Autodesk Inventor part; units mm, degrees
ref_plane "Work Plane2" through (-30, -30, 6) normal (0, 0, -1) x (0, 1, 0)
ref_plane "YZ Plane" through (0, 0, 0) normal (1, 0, 0) x (0, 1, 0)
ref_plane "XZ Plane" through (0, 0, 0) normal (0, 1, 0) x (-1, 0, 0)
ref_plane "Work Plane1" through (0, 0, 0) normal (0, 0, 1) x (1, 0, 0)
ref_plane "Work Plane2" through (-30, -30, 6) normal (0, 0, -1) x (0, 1, 0)
sketch "Sketch1" plane through (0, 0, 0) normal (0, 0, 1) x (1, 0, 0)
  circle A0 centre (-25, 0) radius 1.95
  circle A1 centre (0, -25) radius 1.95
  circle A2 centre (25, -25) radius 1.95
  circle A3 centre (-25, 25) radius 1.95
  circle A4 centre (25, 25) radius 1.95
  circle A5 centre (-25, -25) radius 1.95
  circle A6 centre (0, 25) radius 1.95
  circle A7 centre (25, 0) radius 1.95
  line L0 (-30, -28) -> (-28, -30)
  line L1 (-28, -30) -> (28, -30)
  line L2 (28, -30) -> (30, -28)
  line L3 (30, -28) -> (30, 28)
  line L4 (30, 28) -> (28, 30)
  line L5 (28, 30) -> (-28, 30)
  line L6 (-28, 30) -> (-30, 28)
  line L7 (-30, 28) -> (-30, -28)
  line L8 (43, -44) -> (44, -44)
  line L9 (76, -44) -> (145, -44) construction
  point P0 (0, 0)
  point P1 (30, 25)
extrude "Extrusion1" add sketch "Sketch1" along normal up to surface (6 mm away) contours A0 | A1 | A2 | A3 | A4 | A5 | A6 | A7 | L7 L6 L5 L4 L3 L2 L1 L0
sketch "Sketch2" plane through (-28, 30, 6) normal (0, 0, 1) x (1, 0, 0)
  circle A0 centre (10.5, -12.5) radius 1.95
  circle A1 centre (10.5, -47.5) radius 1.95
  circle A2 centre (45.5, -47.5) radius 1.95
  circle A3 centre (45.5, -12.5) radius 1.95
  point P0 (28, -30)
hole "Hole1" at (-17.5, -17.5, 6) at (17.5, -17.5, 6) at (17.5, 17.5, 6) at (-17.5, 17.5, 6) direction (0, 0, -1) diameter 4 end through all counterbore diameter 8 counterbore depth 4.5
sketch "Sketch10" plane through (0, 0, 0) normal (0, 0, -1) x (-1, 0, 0)
  circle A0 centre (-25, 25) radius 2.325
  circle A1 centre (-25, -25) radius 2.325
  circle A2 centre (25, 25) radius 2.325
  circle A3 centre (25, -25) radius 2.325
  circle A4 centre (25, -25) radius 2.325
  point P0 (0, 0)
hole "Hole3" at (-25, 25, 0) at (25, 25, 0) at (-25, -25, 0) at (25, -25, 0) direction (0, 0, 1) diameter 3.8 depth 20 tip angle 118
sketch "Skizze13" plane through (30, -28, 0) normal (1, 0, 0) x (0, 0, -1)
  line L0 (0, 56) -> (-6, 56)
  line L1 (-6, 56) -> (-6, 58)
  line L2 (0, 56) -> (0, 58)
  line L3 (0, 58) -> (-6, 58)
  line L4 (-6, 58) -> (-6, 63)
  line L5 (-6, 63) -> (6.4834, 75.4834)
  line L6 (10.5521, 75.4834) -> (12.5521, 75.4834)
  line L7 (0, 58) -> (0, 61)
  line L8 (0, 61) -> (8.4834, 69.4834)
  line L9 (8.4834, 69.4834) -> (42.5521, 69.4834)
  line L10 (42.5521, 69.4834) -> (42.5521, 75.4834)
  line L11 (42.5521, 75.4834) -> (6.4834, 75.4834)
  line L12 (42.5521, 75.4834) -> (42.5521, 107.4834)
  point P0 (0, 28)
  dimension "d43" = 5
  dimension "d44" = 135
  dimension "d45" = 135
  dimension "d46" = 0
  dimension "d49" = 6
extrude "Extrusion10" add sketch "Skizze13" against normal up to surface (60 mm away)
ref_plane "Arbeitsebene4" through (-30, 57.7593, -26.2973) normal (1, 0, 0) x (0, -0.9086751, 0.417504)
sketch "Skizze14" plane through (-30, -28, 0) normal (-1, 0, 0) x (0, 0, 1)
  circle A0 centre (-16.0521, 80.4834) radius 1
  circle A1 centre (-31.5521, 101.9834) radius 1
  circle A2 centre (-36.5521, 73.9834) radius 1
  line L0 (-6.4834, 75.4834) -> (-42.5521, 75.4834)
  line L1 (-42.5521, 69.4834) -> (-42.5521, 75.4834)
  line L2 (-42.5521, 75.4834) -> (-12.5521, 75.4834)
  line L3 (-12.5521, 75.4834) -> (-12.5521, 105.4834)
  line L4 (-12.5521, 105.4834) -> (-42.5521, 105.4834)
  line L5 (-42.5521, 105.4834) -> (-42.5521, 75.4834)
  circle A3 centre (-26.5521, 91.4834) radius 2.6486
  line L6 (-34.0521, 83.9834) -> (-19.0521, 83.9834)
  line L7 (-19.0521, 83.9834) -> (-19.0521, 98.9834)
  line L8 (-19.0521, 98.9834) -> (-34.0521, 98.9834)
  line L9 (-34.0521, 98.9834) -> (-34.0521, 83.9834)
  line L10 (-34.0521, 83.9834) -> (-19.0521, 98.9834) construction
  line L11 (-19.0521, 83.9834) -> (-34.0521, 98.9834) construction
  point P0 (0, 28)
  point P1 (-12.5521, 75.4834)
  dimension "d50" = 30
  dimension "d51" = 30
  dimension "d52" = 15
  dimension "d53" = 15
extrude "Extrusion11" add sketch "Skizze14" against normal blind 5 contours L0 L5 L4 L3
sketch "Skizze15" plane through (30, 47.4834, -6.4834) normal (0, 1, 0) x (1, 0, 0)
  circle A0 centre (-15, 20.0687) radius 1.4
  line L0 (2.6067, 20.0687) -> (-28.3951, 20.0687) construction
  line L1 (2.6067, 21.6687) -> (-28.3951, 21.6687)
  line L2 (-28.3951, 18.4687) -> (2.6067, 18.4687)
  arc A1 (2.6067, 18.4687) -> (2.6067, 21.6687) centre (2.6067, 20.0687) ccw
  arc A2 (-28.3951, 21.6687) -> (-28.3951, 18.4687) centre (-28.3951, 20.0687) ccw
  point P0 (-30, -6.4834)
  point P1 (-12.8942, 20.0687)
  dimension "d56" = 3.2
extrude "Extrusion12" cut sketch "Skizze15" against normal through all contours A0 | A1 L2 A2 L1
sketch "Skizze16" plane through (-30, -28, 0) normal (-1, 0, 0) x (0, 0, 1)
  circle A0 centre (-16.0521, 80.4834) radius 1
  circle A1 centre (-31.5521, 101.9834) radius 1
  circle A2 centre (-36.5521, 73.9834) radius 1
  point P0 (0, 28)
extrude "Extrusion13" cut sketch "Skizze16" against normal blind 10
sketch "Skizze17" plane through (-30, 47.4834, -6.4834) normal (0, 1, 0) x (1, 0, 0)
  arc A0 (31.6049, 21.6687) -> (31.6049, 18.4687) centre (31.6049, 20.0687) ccw
  line L0 (44.28, 10.0687) -> (26.9595, 20.0687)
  line L1 (26.9595, 20.0687) -> (44.28, 30.0687)
  line L2 (44.28, 30.0687) -> (44.28, 10.0687)
  line L3 (0, 6.0687) -> (0, 36.0687)
  point P0 (30, -6.4834)
  point P1 (38.5065, 20.0687)
  dimension "d61" = 20
hole "Bohrung4" at (14.28, 47.4834, -16.5521) at (-3.0405, 47.4834, -26.5521) at (14.28, 47.4834, -36.5521) direction (0, -1, 0) diameter 2.8 depth 20 tip angle 118
properties part number "cellSTORM_v5_laserstage"
Could you check a few things on this model? Use its own coordinates, in mm. A direction names the side the tool comes from. Coordinates: 2 decimals unless noted, no trailing zeros. Loops run counter-clockwise (first coordinate to the right, second up) from the corner with the lowest first, then second, coordinate; pieces in that order, holes last.
1) Imagine slicing it at A-A (y = -17.5). List the corners of the cut face in (x, z) for me.
Reported:
outline: (-30, 0) - (-19.5, 0) - (-19.5, 1.5) - (-21.5, 1.5) - (-21.5, 6) - (-30, 6) - close; (-15.5, 0) - (15.5, 0) - (15.5, 1.5) - (13.5, 1.5) - (13.5, 6) - (-13.5, 6) - (-13.5, 1.5) - (-15.5, 1.5) - close; (19.5, 0) - (30, 0) - (30, 6) - (21.5, 6) - (21.5, 1.5) - (19.5, 1.5) - close
2) Which directions (+Z, -Z, +X, -X, +Y, -Y) give clear straight access to the entire face, cutting with the end or side of a thin tool? Please do faces 5 (the face through (-15.8, 15.8, 1.5)), 6 (the face through (-28, 70.983, -26)), 7 (the face through (-28, 62, -12.552)), 8 (the face through (-30, 45, -18)).
Reported:
face 5: +Z
face 6: +X, -X
face 7: +Z, +X, -X, +Y
face 8: +Z, -Z, -X, +Y, -Y
3) Imagine slicing it at D-D (y = 62). List the corners of the cut face in (x, z) for me.
Reported:
outline: (-30, -42.55) - (-25, -42.55) - (-25, -34.05) - (-30, -34.05) - close; (-30, -19.05) - (-25, -19.05) - (-25, -12.55) - (-30, -12.55) - close
4) Thinking about a two-plate mould opening in Y: for faces 1 (the face through (30, 44, -35)), 2 (the face through (15.517, -17.24, 0.74)), 3 (the face through (0, 41, 0)), 4 (the face through (14.8, -14.55, 3.72)), which applies, released by +Y, released by -Y, zero draft, split by the parting line, or undercut?
Reported:
face 1: zero draft
face 2: undercut
face 3: released by +Y
face 4: undercut
5) Imagine slicing it at C-C (x = -17.5). List the corners of the cut face in (y, z) for me, and give its area (3 significant figures).
Reported:
outline: (-30, 0) - (-19.5, 0) - (-19.5, 1.5) - (-21.5, 1.5) - (-21.5, 6) - (-30, 6) - close; (-15.5, 0) - (15.5, 0) - (15.5, 1.5) - (13.5, 1.5) - (13.5, 6) - (-13.5, 6) - (-13.5, 1.5) - (-15.5, 1.5) - close; (19.5, 0) - (33, 0) - (41.48, -8.48) - (41.48, -42.55) - (47.48, -42.55) - (47.48, -6.48) - (35, 6) - (21.5, 6) - (21.5, 1.5) - (19.5, 1.5) - close
area: 594 mm2
6) Will these pins go through, and if not, where does the flat tip stop? pin 1 Ø10 at (x, z) = (23, -28.5) entering from +Y; pin 2 Ø2.5 at (x, z) = (-26.5, -24.5) entering from -Y; pin 3 Ø1.8 at (y, z) = (45.98, -36.55) entering from -X.
Reported:
pin 1: stops at y = 47.48
pin 2: stops at y = 41.48
pin 3: stops at x = -20
7) Imagine slicing it at B-B (x = 25). List the corners of the cut face in (y, z) for me, and give its area (3 significant figures).
Reported:
outline: (-30, 0) - (-26.9, 0) - (-26.9, 6) - (-30, 6) - close; (-23.1, 0) - (23.1, 0) - (23.1, 6) - (-23.1, 6) - close; (26.9, 0) - (33, 0) - (41.48, -8.48) - (41.48, -24.95) - (47.48, -24.95) - (47.48, -6.48) - (35, 6) - (26.9, 6) - close; (41.48, -42.55) - (47.48, -42.55) - (47.48, -28.15) - (41.48, -28.15) - close
area: 613 mm2
8) Please list where these lines run through material, in increasing order: line 1 along X through (y, z) = (17.5, 0.75); line 2 along X through (y, z) = (-25, 3.1); line 3 along Y through (x, z) = (-25, 1.5).
Reported:
line 1: x = -30 to -19.5, -15.5 to 15.5, 19.5 to 30
line 2: x = -30 to -26.9, -23.1 to 23.1, 26.9 to 30
line 3: y = -30 to -26.9, -23.1 to 23.1, 26.9 to 39.5
